Could you check a few things on this model? Use its own coordinates, in mm. Coordinates: 2 decimals unless noted, no trailing zeros. Write each loop counter-clockwise with the first axis right and the second up, starting at its lowest first coordinate (ties: lowest second). Pieces come first, ordered by that corner, then holes.
Item 1: I want a section at B-B on z = 0. Please give me the cut outline in (x, y).
Item 2: I want a section at C-C on x = 45. Please give me the cut outline in (y, z), then the cut area to 3 significant figures.
Item 3: I want a section at A-A on y = 4.4. State how many separate pieces and enclosed holes the cut face has, then the cut area to 3 significant figures.
Item 4: If I drill on probe 1 along Z at (x, y) = (-45, 2.65); probe 2 along X at (y, z) = (1.55, 13.5); probe 3 along X at (y, z) = (3.5, 17), over which ranges is the centre line in solid material (lowest first)?
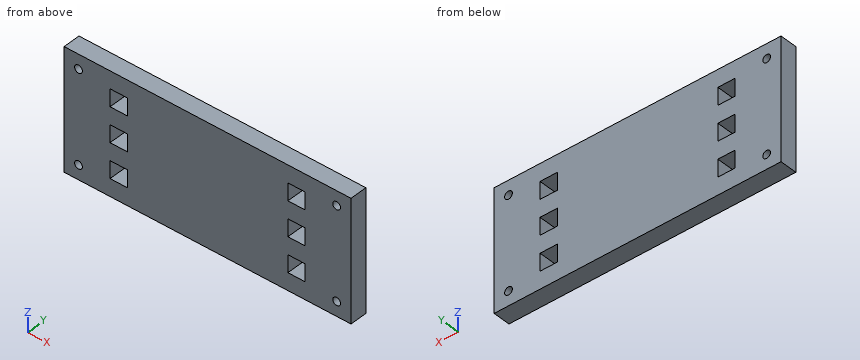
from build123d import *

# Parameters (mm, degrees)
SKETCH2_W           = 100
SKETCH2_H           = 42
SKETCH2_R           = 1.35
SKETCH2_W_2         = 6
SKETCH2_H_2         = 6
BOSS_EXTRUDE1_DEPTH = 6


with BuildPart() as part:
    # Sketch2 → Boss-Extrude1 (new body)
    with BuildSketch(Plane(origin=(0, 0, 0), x_dir=(1, 0, 0), z_dir=(0, 1, 0))):
        Rectangle(SKETCH2_W, SKETCH2_H)
        with Locations((-45, -16)):
            Circle(SKETCH2_R, mode=Mode.SUBTRACT)
        with Locations((-45, 16)):
            Circle(SKETCH2_R, mode=Mode.SUBTRACT)
        with Locations((45, 16)):
            Circle(SKETCH2_R, mode=Mode.SUBTRACT)
        with Locations((45, -16)):
            Circle(SKETCH2_R, mode=Mode.SUBTRACT)
        with Locations((-31, -12)):
            Rectangle(SKETCH2_W_2, SKETCH2_H_2, mode=Mode.SUBTRACT)
        with Locations((-31, 0)):
            Rectangle(SKETCH2_W_2, SKETCH2_H_2, mode=Mode.SUBTRACT)
        with Locations((-31, 12)):
            Rectangle(SKETCH2_W_2, SKETCH2_H_2, mode=Mode.SUBTRACT)
        with Locations((31, -12)):
            Rectangle(SKETCH2_W_2, SKETCH2_H_2, mode=Mode.SUBTRACT)
        with Locations((31, 0)):
            Rectangle(SKETCH2_W_2, SKETCH2_H_2, mode=Mode.SUBTRACT)
        with Locations((31, 12)):
            Rectangle(SKETCH2_W_2, SKETCH2_H_2, mode=Mode.SUBTRACT)
    extrude(amount=BOSS_EXTRUDE1_DEPTH)


solid = part.part
Response values:
1. outline: (-50, 0) - (-34, 0) - (-34, 6) - (-50, 6) - close; (-28, 0) - (28, 0) - (28, 6) - (-28, 6) - close; (34, 0) - (50, 0) - (50, 6) - (34, 6) - close
2. outline: (0, -21) - (6, -21) - (6, -17.35) - (0, -17.35) - close; (0, -14.65) - (6, -14.65) - (6, 14.65) - (0, 14.65) - close; (0, 17.35) - (6, 17.35) - (6, 21) - (0, 21) - close
2. area: 220 mm2
3. separate pieces: 1
3. enclosed holes: 10
3. area: 3,960 mm2
4. probe 1: z = -21 to -17.35, -14.65 to 14.65, 17.35 to 21
4. probe 2: x = -50 to -34, -28 to 28, 34 to 50
4. probe 3: x = -50 to -45.91, -44.09 to 44.09, 45.91 to 50
